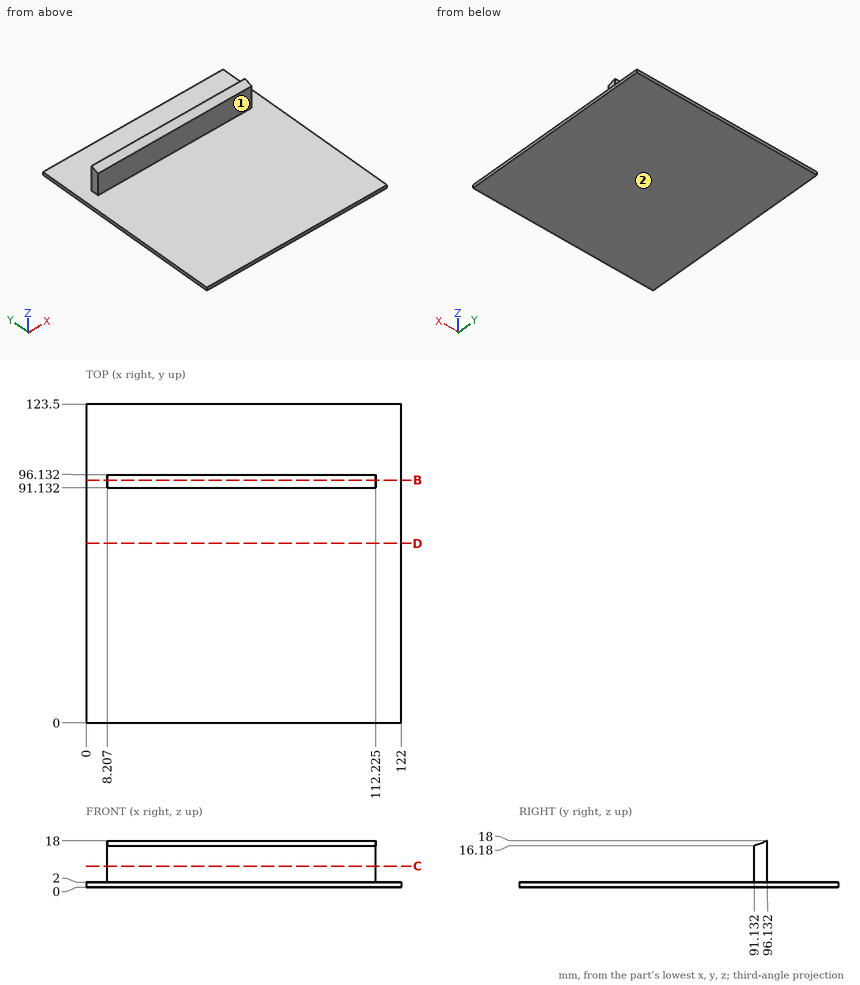
Answer from the drawing. Dimensions are ordinates in mm from the lowest x, y and z of the part. A direction names the side the tool comes from. Coordinates: 2 decimals unless noted, no trailing zeros. Write each loop counter-clockwise with the first axis right and the second up, starting at its lowest first coordinate (ties: lowest second). Pieces come first, ordered by that corner, then holes. Notation, with made-up numbers: M -23,-26.5 L -2,-26.5 A18 cw -2,-1.5 Z; hole C 17,43 d6. An arc over 180 degrees is marked long. Use a Markdown table: item, result.
Q1. Straight lines are drawn through the part: L1, parallel to Z at x = 98, y = 115.5; L2, parallel to Y at x = 65, z = 15.5; L3, parallel to Z at x = 8.5, y = 91.5 (1 decimal). For each, find the intervals that lie inside material, in ascending order. Write a range as [from, to].
Answer block:
| item | result |
|---|---|
| L1 | z = [0, 2] |
| L2 | y = [91.13, 96.13] |
| L3 | z = [0, 16.3] |
Q2. The part is cut by section B-B, the plane y = 94. Write down the section's boundary in (x, z) (1 decimal).
Answer block:
| item | result |
|---|---|
| outline | M 0,0 L 122,0 L 122,2 L 112.2,2 L 112.2,17.2 L 8.2,17.2 L 8.2,2 L 0,2 Z |
Q3. The part is cut by section C-C, the plane z = 8.25. Write down the section's boundary in (x, y) (1 decimal), then the cut area to 3 significant figures.
Answer block:
| item | result |
|---|---|
| outline | M 8.2,91.1 L 112.2,91.1 L 112.2,96.1 L 8.2,96.1 Z |
| area | 520 mm2 |
Q4. Each of these flat-tipped pins is pushed along its axis until it touches: pin 1 Ø5 at (x, z) = (72, 3.5) entering from +Y; pin 2 Ø8 at (x, z) = (38.5, 8) entering from -Y; pin 3 Ø1.5 at (y, z) = (94, 11) entering from +X (1 decimal); pin 4 Ø5.5 at (y, z) = (94.5, 12.5) entering from -X. Where does it stop, or does it pass through?
Answer block:
| item | result |
|---|---|
| pin 1 | stops at y = 123.5 |
| pin 2 | stops at y = 91.13 |
| pin 3 | stops at x = 112.2 |
| pin 4 | stops at x = 8.21 |
Q5. The part is cut by section D-D, the plane y = 69.5. Write down the section's boundary in (x, z).
Answer block:
| item | result |
|---|---|
| outline | M 0,0 L 122,0 L 122,2 L 0,2 Z |
Q6. Which of the six approach directions +Z, -Z, +X, -X, +Y, -Y give full straight-line access (tool end or side, diameter ignored) to the marked faces 1 and 2?
Answer block:
| item | result |
|---|---|
| face 1 | +Z, +X, -X, -Y |
| face 2 | -Z, +X, -X, +Y, -Y |
